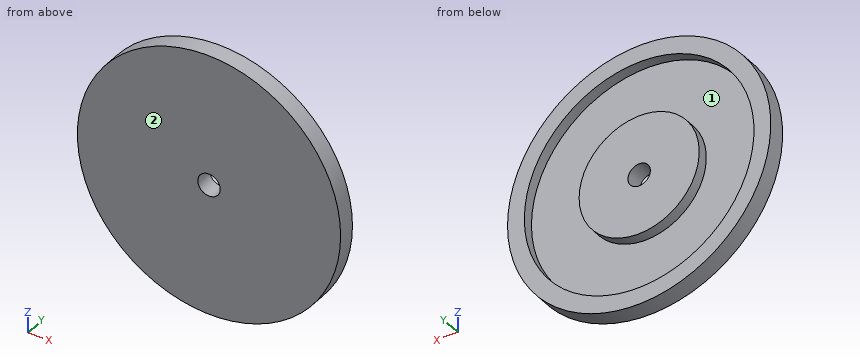
```python
from build123d import *

# Parameters (mm, degrees)
SKETCH016_R     = 34
PAD013_DEPTH    = 6
SKETCH017_R     = 74.5
PAD014_DEPTH    = 4
SKETCH018_R     = 74.5
SKETCH018_R_2   = 65
PAD015_DEPTH    = 6
SKETCH019_R     = 6.35
POCKET003_DEPTH = 10.001


with BuildPart() as part:
    # Sketch016 → Pad013 (new body)
    with BuildSketch(Plane.XZ):
        Circle(SKETCH016_R)
    extrude(amount=PAD013_DEPTH)

    # Sketch017 (on Face3 of Pad013) → Pad014 (join)
    with BuildSketch(Plane.XZ.offset(6)):
        Circle(SKETCH017_R)
    extrude(amount=PAD014_DEPTH)

    # Sketch018 (on Face2 of Pad014) → Pad015 (join)
    with BuildSketch(Plane(origin=(0, -6, 0), x_dir=(1, 0, 0), z_dir=(0, 1, 0))):
        Circle(SKETCH018_R)
        Circle(SKETCH018_R_2, mode=Mode.SUBTRACT)
    extrude(amount=PAD015_DEPTH)

    # Sketch019 (on Face8 of Pad015) → Pocket003 (cut, through all)
    with BuildSketch(Plane(origin=(0, 0, 0), x_dir=(1, 0, 0), z_dir=(0, 1, 0))):
        Circle(SKETCH019_R)
    extrude(amount=-POCKET003_DEPTH, mode=Mode.SUBTRACT)


solid = part.part
```
Geometry: final body of the model. Coordinates: model frame, mm. Face numbers are marked on the shaded views. Round coordinates to 2 decimals unless told otherwise and drop trailing zeros. Order: outer loops, then holes, each group sorted by start corner. A loop starts at its lowest first (then second) coordinate and runs counter-clockwise, first axis right, second up. Notation, with made-up numbers: (87, -7) -> (123, -7) arc R12 ccw to (123, 12) -> close; hole circle Ø10 at (7.25, 10). An arc over 180 degrees is marked (long way). Use one line per item in the form item = value. Start each with the question number.
1. Line query: probe 1 along Z at (x, y) = (0, -2.3); probe 2 along Z at (x, y) = (30.5, -1); probe 3 along Z at (x, y) = (23.5, -2). Output: solid intervals per line, ascending.
2. Pin query (flat end, axial travel): pin 1 Ø4 at (x, y) = (-20.5, -1.5) entering from +Z; pin 2 Ø3 at (x, y) = (-6, -8.5) entering from +Z; pin 3 Ø3 at (x, y) = (1.5, -2) entering from -Z. Return the tip coordinate at first contact, or that it passes through.
3. Cut plane A-A (x = 0). Return the cut outline in (y, z).
4. Cut plane B-B (z = 0). Return the cut outline in (x, y).
5. Cut plane D-D (z = -48.5). Return the cut outline in (x, y), then the cut area to 3 significant figures.
6. Cut plane C-C (x = -29.5). Return the cut outline in (y, z), then the cut area to 3 significant figures.
7. Draft query along X for the marked faces 1 and 2. Return one class per face: pulls with the +X half, pulls with the -X half, needs draft (parallel to the pull), parting line crosses it, or undercut.
Solution:
q1.probe_1 = -74.5 to -65, -34 to -6.35, 6.35 to 34, 65 to 74.5
q1.probe_2 = -67.97 to -57.4, -15.02 to 15.02, 57.4 to 67.97
q1.probe_3 = -70.7 to -60.6, -24.57 to 24.57, 60.6 to 70.7
q2.pin_1 = 72.17
q2.pin_2 = 74.36
q2.pin_3 = -74.5
q3.outline = (-10, -74.5) -> (0, -74.5) -> (0, -65) -> (-6, -65) -> (-6, -34) -> (0, -34) -> (0, -6.35) -> (-10, -6.35) -> close; (-10, 6.35) -> (0, 6.35) -> (0, 34) -> (-6, 34) -> (-6, 65) -> (0, 65) -> (0, 74.5) -> (-10, 74.5) -> close
q4.outline = (-74.5, -10) -> (-6.35, -10) -> (-6.35, 0) -> (-34, 0) -> (-34, -6) -> (-65, -6) -> (-65, 0) -> (-74.5, 0) -> close; (6.35, -10) -> (74.5, -10) -> (74.5, 0) -> (65, 0) -> (65, -6) -> (34, -6) -> (34, 0) -> (6.35, 0) -> close
q5.outline = (-56.55, -10) -> (56.55, -10) -> (56.55, 0) -> (43.28, 0) -> (43.28, -6) -> (-43.28, -6) -> (-43.28, 0) -> (-56.55, 0) -> close
q5.area = 612 mm^2
q6.outline = (-10, -68.41) -> (0, -68.41) -> (0, -57.92) -> (-6, -57.92) -> (-6, -16.9) -> (0, -16.9) -> (0, 16.9) -> (-6, 16.9) -> (-6, 57.92) -> (0, 57.92) -> (0, 68.41) -> (-10, 68.41) -> close
q6.area = 876 mm^2
q7.face_1 = undercut
q7.face_2 = needs draft
